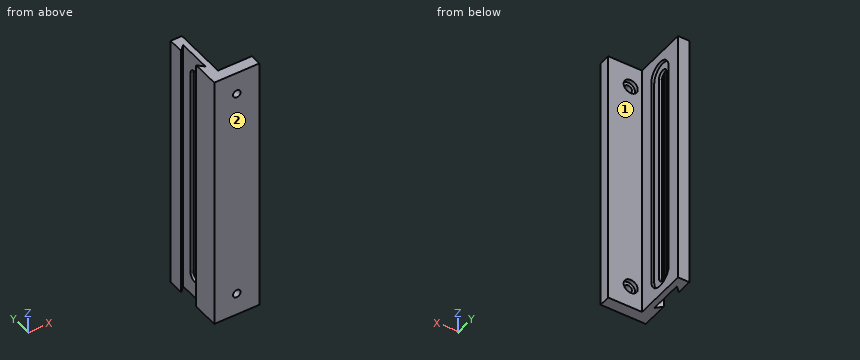
```python
from build123d import *

# Parameters (mm, degrees)
SKETCH1_W                                           = 25.4
SKETCH1_H                                           = 147.32
BOSS_EXTRUDE1_DEPTH                                 = 6.35
SKETCH2_W                                           = 147.32
SKETCH2_H                                           = 30.48
BOSS_EXTRUDE2_DEPTH                                 = 6.35
CBORE_FOR_6_BINDING_HEAD_MACHINE_SCREW1_D           = 4.3053
CBORE_FOR_6_BINDING_HEAD_MACHINE_SCREW1_CBORE_D     = 7.9375
CBORE_FOR_6_BINDING_HEAD_MACHINE_SCREW1_CBORE_DEPTH = 2.2098
CUT_EXTRUDE1_DEPTH                                  = 152.641403647
CUT_EXTRUDE2_DEPTH                                  = 1.5875
CUT_EXTRUDE3_DEPTH                                  = 153.569239364


with BuildPart() as part:
    # Sketch1 → Boss-Extrude1 (new body)
    with BuildSketch(Plane(origin=(0, 0, 0), x_dir=(1, 0, 0), z_dir=(0, 1, 0))):
        with Locations((12.7, 73.66)):
            Rectangle(SKETCH1_W, SKETCH1_H)
    extrude(amount=-BOSS_EXTRUDE1_DEPTH)

    # Sketch2 → Boss-Extrude2 (add)
    with BuildSketch(Plane.ZY):
        with Locations((-73.66, 15.24)):
            Rectangle(SKETCH2_W, SKETCH2_H)
    extrude(amount=-BOSS_EXTRUDE2_DEPTH)

    # CBORE for #6 Binding Head Machine Screw1 (through all)
    with Locations(Plane(origin=(0, 0, 0), x_dir=(1, 0, 0), z_dir=(0, 1, 0))):
        with Locations((12.7, 12.7), (12.7, 134.62)):
            CounterBoreHole(CBORE_FOR_6_BINDING_HEAD_MACHINE_SCREW1_D / 2, CBORE_FOR_6_BINDING_HEAD_MACHINE_SCREW1_CBORE_D / 2, CBORE_FOR_6_BINDING_HEAD_MACHINE_SCREW1_CBORE_DEPTH)

    # Sketch9 → Cut-Extrude1 (cut, through all)
    with BuildSketch(Plane(origin=(6.35, 0, 0), x_dir=(0, 0, -1), z_dir=(1, 0, 0))):
        with BuildLine():
            Line((12.7, 18.415), (134.62, 18.415))
            ThreePointArc((134.62, 18.415), (137.795, 15.24), (134.62, 12.065))
            Line((134.62, 12.065), (12.7, 12.065))
            ThreePointArc((12.7, 12.065), (9.525, 15.24), (12.7, 18.415))
        make_face()
    extrude(amount=-CUT_EXTRUDE1_DEPTH, mode=Mode.SUBTRACT)

    # Sketch12 → Cut-Extrude2 (cut)
    with BuildSketch(Plane(origin=(6.35, 0, 0), x_dir=(0, 0, -1), z_dir=(1, 0, 0))):
        with BuildLine():
            Line((12.7, 22.493732), (134.62, 22.493732))
            ThreePointArc((134.62, 22.493732), (141.873732, 15.24), (134.62, 7.986268))
            Line((134.62, 7.986268), (12.7, 7.986268))
            ThreePointArc((12.7, 7.986268), (5.446268, 15.24), (12.7, 22.493732))
        make_face()
    extrude(amount=-CUT_EXTRUDE2_DEPTH, mode=Mode.SUBTRACT)

    # Sketch13 → Cut-Extrude3 (cut, through all)
    with BuildSketch(Plane(origin=(0, 0, -147.32), x_dir=(-1, 0, 0), z_dir=(0, 0, -1))):
        Polygon((0, 21.59), (0, 8.89), (-3.175, 5.715), (-3.175, 24.765), align=None)
    extrude(amount=-CUT_EXTRUDE3_DEPTH, mode=Mode.SUBTRACT)


solid = part.part
```
For this review, take the finished solid that the model builds, in its own axes (mm). Face numbers are marked on the shaded views. A direction names the side the tool comes from. Coordinates: 2 decimals unless noted, no trailing zeros. Loops run counter-clockwise (first coordinate to the right, second up) from the corner with the lowest first, then second, coordinate; pieces in that order, holes last.
1. For the marked faces 1 and 2, list the 3-axis set-ups (+Z, -Z, +X, -X, +Y, -Y) from which the entire face can be reached by the end or side of a thin tool; tool diameter is ignored.
2. Insertion check: P1, Ø1, axis at x = 22, z = -55, coming from the +Y side; P2, Ø2.5, axis at x = 13, z = -13.5, coming from the +Y side; P3, Ø1.5, axis at y = 10.5, z = -106.5, coming from the +X side; P4, Ø9.5, axis at y = 14, z = -43.5, coming from the -X side (3 decimals). Each pin has a flat end and moves straight along its axis. Give the tip position at first contact, or say it passes through.
3. Add section D-D, the plane x = 21.75. Give the boundary of the cut face in (y, z), then the cut area to 3 significant figures.
4. For line 1 (Z direction, x = 12.7, y = -4.6); line 2 (Z direction, x = 12.7, y = -0.6); line 3 (X direction, y = -3, z = -12), list the stretches that pass through material, from the lowest coordinate up.
5. Add section C-C, the plane x = 12.7. Give the boundary of the cut face in (y, z).
Result:
1. face 1: +Z, -Z, +X, +Y
1. face 2: +Z, -Z, +X, -X, -Y
2. P1: stops at y = 0
2. P2: passes through
2. P3: stops at x = 4.76
2. P4: stops at x = 3.175
3. outline: (-6.35, -147.32) - (0, -147.32) - (0, 0) - (-6.35, 0) - close
3. area: 935 mm2
4. line 1: z = -147.32 to -136.77, -132.47 to -14.85, -10.55 to 0
4. line 2: z = -147.32 to -138.59, -130.65 to -16.67, -8.73 to 0
4. line 3: x = 0 to 10.66, 14.74 to 25.4
5. outline: (-6.35, -147.32) - (0, -147.32) - (0, -138.59) - (-2.21, -138.59) - (-2.21, -136.77) - (-6.35, -136.77) - close; (-6.35, -132.47) - (-2.21, -132.47) - (-2.21, -130.65) - (0, -130.65) - (0, -16.67) - (-2.21, -16.67) - (-2.21, -14.85) - (-6.35, -14.85) - close; (-6.35, -10.55) - (-2.21, -10.55) - (-2.21, -8.73) - (0, -8.73) - (0, 0) - (-6.35, 0) - close
